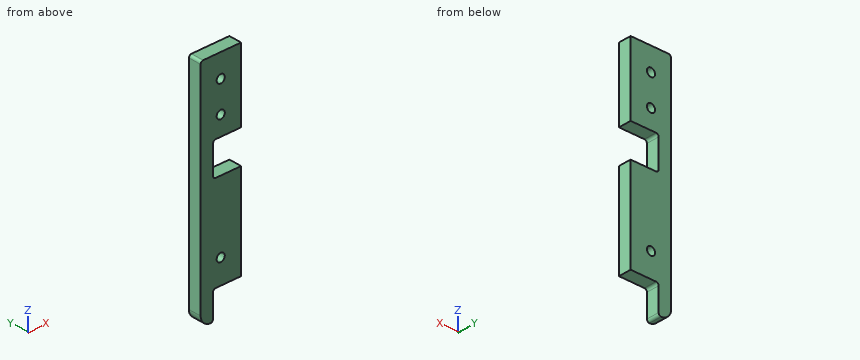
Autodesk Inventor part; units mm, degrees
ref_plane "YZ Plane" through (0, 0, 0) normal (1, 0, 0) x (0, 1, 0)
ref_plane "XZ Plane" through (0, 0, 0) normal (0, 1, 0) x (-1, 0, 0)
ref_plane "XY Plane" through (0, 0, 0) normal (0, 0, 1) x (1, 0, 0)
sketch "Sketch1" plane through (0, 0, 0) normal (0, 1, 0) x (-1, 0, 0)
  line L0 (0, 0) -> (15.9, 0)
  line L1 (15.9, -16) -> (15.9, -100.5)
  line L2 (10, -104.5) -> (0, -104.5)
  line L3 (0, -104.5) -> (0, 0)
  line L4 (0, -104.5) -> (11, -104.5)
  line L5 (11, -103.5) -> (11, -94.5)
  line L6 (10, -93.5) -> (0, -93.5)
  line L7 (0, -93.5) -> (0, -104.5)
  line L8 (10, -43.5) -> (0, -43.5)
  line L9 (0, -43.5) -> (0, -56.5)
  line L10 (0, -56.5) -> (10, -56.5)
  line L11 (11, -55.5) -> (11, -44.5)
  line L12 (15.9, 0) -> (0, 0)
  line L13 (0, 0) -> (0, -15)
  line L14 (0, -15) -> (14.9, -15)
  line L15 (15.9, -15) -> (15.9, 0)
  arc A0 (11.9, -104.5) -> (15.9, -100.5) centre (11.9, -100.5) ccw
  arc A1 (15.9, -16) -> (14.9, -15) centre (14.9, -16) ccw
  arc A2 (11, -44.5) -> (10, -43.5) centre (10, -44.5) ccw
  arc A3 (10, -56.5) -> (11, -55.5) centre (10, -55.5) ccw
  arc A4 (11, -94.5) -> (10, -93.5) centre (10, -94.5) ccw
  line L16 (11.9, -104.5) -> (12, -104.5)
  arc A5 (11, -103.5) -> (12, -104.5) centre (12, -103.5) ccw
  point P0 (15.9, -104.5)
  point P1 (11, -93.5)
  point P2 (11, -43.5)
  point P3 (11, -56.5)
  point P4 (0, -43.5)
  point P5 (0, -56.5)
  point P6 (11.9667, -104.4994)
  dimension "d0" = 15.9
  dimension "d1" = 104.5
  dimension "d2" = 11
  dimension "d3" = 11
  dimension "d4" = 11
  dimension "d5" = 13
  dimension "d6" = 56.5
  dimension "d7" = 15
  dimension "d8" = 4
  dimension "d9" = 1
  dimension "d22" = 1
extrude "Extrusion1" add sketch "Sketch1" along normal blind 5 contours L1 A0 A5 L5 A4 L6 L3 L10 A3 L11 A2 L8 L14 A1
sketch "Sketch2" plane through (0, 5, 0) normal (0, 1, 0) x (1, 0, 0)
  line L0 (-8, -6.918) -> (-8, 116.4057) construction
  line L1 (0, 15) -> (0, 43.5) construction
  point P0 (0, 0)
  point P1 (-8, 84)
  point P2 (-8, 36)
  point P3 (-8, 24)
  dimension "d12" = 8
  dimension "d13" = 36
  dimension "d14" = 84
  dimension "d23" = 24
hole "Hole1" at (-8, 5, -84) at (-8, 5, -36) at (-8, 5, -24) direction (0, -1, 0) diameter 3.2 end through all
properties part number "Lower slide"
Source: CAD feature listing. Evaluate the final solid. Frame: model axes, mm. Round coordinates to 2 decimals unless told otherwise and drop trailing zeros. Loops run counter-clockwise (first coordinate to the right, second up) from the corner with the lowest first, then second, coordinate; pieces in that order, holes last. Notation, with made-up numbers: M 26.5,-2 L 47.5,-2 A8 ccw 47.5,3 Z; hole C -30.5,55.25 d4. An arc over 180 degrees is marked long. Use a Markdown table: item, result. Add a question column.
1. Contact query for flat-ended pins moving along their axis: pin 1 (5 mm diameter, centred on x = -8, z = -55, fed in from +Y); pin 2 (1.5 mm diameter, centred on y = 3, z = -99.5, fed in from +X); pin 3 (5 mm diameter, centred on x = -6, z = -48, fed in from -Y). Output: stop coordinate, or through.
2. Cut plane A-A, the plane z = -24. Output: boundary loops of the cut face in (x, y).
3. Cut plane C-C, the plane y = 2.3. Output: boundary loops of the cut face in (x, z).
4. Cut plane D-D, the plane z = -51.5. Output: boundary loops of the cut face in (x, y).
5. Cut plane B-B, the plane x = -8. Output: boundary loops of the cut face in (y, z).
6. Ray query, line 1 along Z through (x, y) = (-8, 1); line 2 along X through (y, z) = (2.2, -36); line 3 along Z through (x, y) = (-10, 4.3). Return the intervals inside material, ascending. Write a range as [from, to].
Solution:
| question | item | result |
|---|---|---|
| 1 | pin 1 | stops at y = 5 |
| 1 | pin 2 | stops at x = -11 |
| 1 | pin 3 | passes through |
| 2 | outline | M -15.9,0 L -9.6,0 L -9.6,5 L -15.9,5 Z; M -6.4,0 L 0,0 L 0,5 L -6.4,5 Z |
| 3 | outline | M -15.9,-100.5 A4 ccw -12,-104.5 A1 ccw -11,-103.5 L -11,-94.5 A1 cw -10,-93.5 L 0,-93.5 L 0,-56.5 L -10,-56.5 A1 cw -11,-55.5 L -11,-44.5 A1 cw -10,-43.5 L 0,-43.5 L 0,-15 L -14.9,-15 A1 ccw -15.9,-16 Z; hole C -8,-84 d3.2; hole C -8,-36 d3.2; hole C -8,-24 d3.2 |
| 4 | outline | M -15.9,0 L -11,0 L -11,5 L -15.9,5 Z |
| 5 | outline | M 0,-93.5 L 5,-93.5 L 5,-85.6 L 0,-85.6 Z; M 0,-82.4 L 5,-82.4 L 5,-56.5 L 0,-56.5 Z; M 0,-43.5 L 5,-43.5 L 5,-37.6 L 0,-37.6 Z; M 0,-34.4 L 5,-34.4 L 5,-25.6 L 0,-25.6 Z; M 0,-22.4 L 5,-22.4 L 5,-15 L 0,-15 Z |
| 6 | line 1 | z = [-93.5, -85.6], [-82.4, -56.5], [-43.5, -37.6], [-34.4, -25.6], [-22.4, -15] |
| 6 | line 2 | x = [-15.9, -9.6], [-6.4, 0] |
| 6 | line 3 | z = [-93.5, -56.5], [-43.5, -15] |
